Geometry: final body of the model. Coordinates: model frame, mm. Give positions to 0.01 mm unless a question says otherwise; leave off trailing zeros.
from build123d import *

# Parameters (mm, degrees)
SKETCH1_R           = 1.5
BOSS_EXTRUDE1_DEPTH = 2.54
SKETCH3_W           = 31.262195004
SKETCH3_H           = 33.538767861
SKETCH3_W_2         = 23.950407972
SKETCH3_H_2         = 32.282278018
SKETCH3_W_3         = 37.965776447
SKETCH3_H_3         = 40.338637474
SKETCH3_W_4         = 25.395042547
SKETCH3_H_4         = 35.871060739
SKETCH3_W_5         = 33.559034537
SKETCH3_W_6         = 22.639264221
SKETCH3_R           = 1.5
CUT_EXTRUDE1_DEPTH  = 2.54
SKETCH4_W           = 37.965776447
SKETCH4_H           = 14.057244835
SKETCH4_W_2         = 33.559034537
BOSS_EXTRUDE2_DEPTH = 2.54


with BuildPart() as part:
    # Sketch1 → Boss-Extrude1 (new body)
    with BuildSketch(Plane(origin=(0, 0, 0), x_dir=(1, 0, 0), z_dir=(0, 1, 0))):
        Polygon((86.436432638, 72.445920304), (-59.563567362, 72.445920304), (-59.563567362, -123.554079696), (-39.563567362, -137.554079696), (66.436432638, -137.554079696), (86.436432638, -123.554079696), align=None)
        with Locations((-49.563567362, -120.554079696)):
            Circle(SKETCH1_R, mode=Mode.SUBTRACT)
        with Locations((-39.563567362, -120.554079696)):
            Circle(SKETCH1_R, mode=Mode.SUBTRACT)
        with Locations((-29.563567362, -120.554079696)):
            Circle(SKETCH1_R, mode=Mode.SUBTRACT)
        with Locations((-49.563567362, -92.554079696)):
            Circle(SKETCH1_R, mode=Mode.SUBTRACT)
        with Locations((-39.563567362, -92.554079696)):
            Circle(SKETCH1_R, mode=Mode.SUBTRACT)
        with Locations((-29.563567362, -92.554079696)):
            Circle(SKETCH1_R, mode=Mode.SUBTRACT)
        with Locations((-6.563567362, -86.554079696)):
            Circle(SKETCH1_R, mode=Mode.SUBTRACT)
        with Locations((-39.563567362, -37.554079696)):
            Circle(SKETCH1_R, mode=Mode.SUBTRACT)
        with Locations((-29.563567362, -37.554079696)):
            Circle(SKETCH1_R, mode=Mode.SUBTRACT)
        with Locations((-6.563567362, -46.554079696)):
            Circle(SKETCH1_R, mode=Mode.SUBTRACT)
        with Locations((-6.563567362, -38.554079696)):
            Circle(SKETCH1_R, mode=Mode.SUBTRACT)
        with Locations((33.436432638, -86.554079696)):
            Circle(SKETCH1_R, mode=Mode.SUBTRACT)
        with Locations((56.436432638, -120.554079696)):
            Circle(SKETCH1_R, mode=Mode.SUBTRACT)
        with Locations((66.436432638, -120.554079696)):
            Circle(SKETCH1_R, mode=Mode.SUBTRACT)
        with Locations((76.436432638, -120.554079696)):
            Circle(SKETCH1_R, mode=Mode.SUBTRACT)
        with Locations((56.436432638, -92.554079696)):
            Circle(SKETCH1_R, mode=Mode.SUBTRACT)
        with Locations((66.436432638, -92.554079696)):
            Circle(SKETCH1_R, mode=Mode.SUBTRACT)
        with Locations((76.436432638, -92.554079696)):
            Circle(SKETCH1_R, mode=Mode.SUBTRACT)
        with Locations((33.436432638, -46.554079696)):
            Circle(SKETCH1_R, mode=Mode.SUBTRACT)
        with Locations((33.436432638, -38.554079696)):
            Circle(SKETCH1_R, mode=Mode.SUBTRACT)
        with Locations((56.436432638, -37.554079696)):
            Circle(SKETCH1_R, mode=Mode.SUBTRACT)
        with Locations((66.436432638, -37.554079696)):
            Circle(SKETCH1_R, mode=Mode.SUBTRACT)
        with Locations((-39.563567362, -17.554079696)):
            Circle(SKETCH1_R, mode=Mode.SUBTRACT)
        with Locations((-29.563567362, -17.554079696)):
            Circle(SKETCH1_R, mode=Mode.SUBTRACT)
        with Locations((-13.813567362, -26.554079696)):
            Circle(SKETCH1_R, mode=Mode.SUBTRACT)
        with Locations((-19.813567362, -0.554079696)):
            Circle(SKETCH1_R, mode=Mode.SUBTRACT)
        with Locations((-6.563567362, 12.445920304)):
            Circle(SKETCH1_R, mode=Mode.SUBTRACT)
        with Locations((-39.563567362, 32.445920304)):
            Circle(SKETCH1_R, mode=Mode.SUBTRACT)
        with Locations((-29.563567362, 32.445920304)):
            Circle(SKETCH1_R, mode=Mode.SUBTRACT)
        with Locations((-39.563567362, 52.445920304)):
            Circle(SKETCH1_R, mode=Mode.SUBTRACT)
        with Locations((-29.563567362, 52.445920304)):
            Circle(SKETCH1_R, mode=Mode.SUBTRACT)
        with Locations((-21.563567362, 27.445920304)):
            Circle(SKETCH1_R, mode=Mode.SUBTRACT)
        with Locations((-6.563567362, 52.445920304)):
            Circle(SKETCH1_R, mode=Mode.SUBTRACT)
        with Locations((-6.563567362, 60.445920304)):
            Circle(SKETCH1_R, mode=Mode.SUBTRACT)
        with Locations((40.686432638, -26.554079696)):
            Circle(SKETCH1_R, mode=Mode.SUBTRACT)
        with Locations((46.686432638, -0.554079696)):
            Circle(SKETCH1_R, mode=Mode.SUBTRACT)
        with Locations((33.436432638, 12.445920304)):
            Circle(SKETCH1_R, mode=Mode.SUBTRACT)
        with Locations((56.436432638, -17.554079696)):
            Circle(SKETCH1_R, mode=Mode.SUBTRACT)
        with Locations((66.436432638, -17.554079696)):
            Circle(SKETCH1_R, mode=Mode.SUBTRACT)
        with Locations((48.436432638, 27.445920304)):
            Circle(SKETCH1_R, mode=Mode.SUBTRACT)
        with Locations((33.436432638, 52.445920304)):
            Circle(SKETCH1_R, mode=Mode.SUBTRACT)
        with Locations((33.436432638, 60.445920304)):
            Circle(SKETCH1_R, mode=Mode.SUBTRACT)
        with Locations((56.436432638, 32.445920304)):
            Circle(SKETCH1_R, mode=Mode.SUBTRACT)
        with Locations((66.436432638, 32.445920304)):
            Circle(SKETCH1_R, mode=Mode.SUBTRACT)
        with Locations((56.436432638, 52.445920304)):
            Circle(SKETCH1_R, mode=Mode.SUBTRACT)
        with Locations((66.436432638, 52.445920304)):
            Circle(SKETCH1_R, mode=Mode.SUBTRACT)
    extrude(amount=BOSS_EXTRUDE1_DEPTH)

    # Sketch3 → Cut-Extrude1 (cut)
    with BuildSketch(Plane(origin=(0, 2.54, 0), x_dir=(1, 0, 0), z_dir=(0, 1, 0))):
        with Locations((13.218035303, 32.06539189)):
            Rectangle(SKETCH3_W, SKETCH3_H)
        with Locations((-40.771807944, 7.158059835)):
            Rectangle(SKETCH3_W_2, SKETCH3_H_2)
        with Locations((-33.764123707, -66.570477409)):
            Rectangle(SKETCH3_W_3, SKETCH3_H_3)
        with Locations((14.037654844, -68.804265777)):
            Rectangle(SKETCH3_W_4, SKETCH3_H_4)
        with Locations((63.014708218, -66.570477409)):
            Rectangle(SKETCH3_W_5, SKETCH3_H_3)
        with Locations((68.474593376, 7.158059835)):
            Rectangle(SKETCH3_W_6, SKETCH3_H_2)
        with Locations((3.209707255, -16.593217859)):
            Circle(SKETCH3_R)
        with Locations((12.713373484, -28.278053387)):
            Circle(SKETCH3_R)
        with Locations((21.593848485, -16.593217859)):
            Circle(SKETCH3_R)
        with Locations((8.479175475, 0)):
            Circle(SKETCH3_R)
        with Locations((-2.413062199, -113.470581074)):
            Circle(SKETCH3_R)
        with Locations((8.479175475, -113.470581074)):
            Circle(SKETCH3_R)
        with Locations((19.509289574, -113.470581074)):
            Circle(SKETCH3_R)
        with Locations((19.509289574, -122.554079696)):
            Circle(SKETCH3_R)
        with Locations((-2.413062199, -122.554079696)):
            Circle(SKETCH3_R)
        with Locations((8.479175475, -122.554079696)):
            Circle(SKETCH3_R)
        with Locations((8.479175475, -132.554079696)):
            Circle(SKETCH3_R)
        with Locations((-2.413062199, -132.554079696)):
            Circle(SKETCH3_R)
        with Locations((19.509289574, -132.554079696)):
            Circle(SKETCH3_R)
    extrude(amount=-CUT_EXTRUDE1_DEPTH, mode=Mode.SUBTRACT)

    # Sketch4 → Boss-Extrude2 (add)
    with BuildSketch(Plane(origin=(0, 0, 0), x_dir=(1, 0, 0), z_dir=(0, 1, 0))):
        with Locations((-33.764123707, -66.965043616)):
            Rectangle(SKETCH4_W, SKETCH4_H)
        with Locations((63.014708218, -66.965043616)):
            Rectangle(SKETCH4_W_2, SKETCH4_H)
    extrude(amount=BOSS_EXTRUDE2_DEPTH)


solid = part.part
Item 1: Pin query (flat end, axial travel): pin 1 (1 mm diameter, centred on x = -22.5, z = 45.5, fed in from -Y); pin 2 (0.8 mm diameter, centred on x = -40, y = 2, fed in from +Z); pin 3 (0.8 mm diameter, centred on x = -42.5, y = 1.5, fed in from +Z); pin 4 (1.8 mm diameter, centred on x = 66.44, z = 37.55, fed in from +Y). Return the tip coordinate at first contact, or that it passes through.
Values follow:
pin 1: stops at y = 0
pin 2: stops at z = 137.53
pin 3: stops at z = 135.78
pin 4: passes through
Item 2: Ray query, probe 1 along X at (y, z) = (2.4, 53); probe 2 along Z at (x, y) = (-25, 1.95); probe 3 along X at (y, z) = (1.85, 4). Return the intervals inside material, ascending.
Values follow:
probe 1: x = -59.56 to -52.75, -14.78 to 1.34, 26.74 to 46.24, 79.79 to 86.44
probe 2: z = -72.45 to 46.4, 59.94 to 73.99, 86.74 to 137.55
probe 3: x = -59.56 to -52.75, -28.8 to 57.15, 79.79 to 86.44
Item 3: Section query A-A on y = 0.6. Give the number of separate pieces and of enclosed holes in the cut face, plus the area to 3 significant figures.
Values follow:
separate pieces: 1
enclosed holes: 67
area: 24,600 mm2
